Could you check a few things on this model? Use its own coordinates, in mm. A direction names the side the tool comes from. Give positions to 0.01 mm unless a question says otherwise; leave off trailing zeros. Order: outer loops, then holes, each group sorted by start corner. A loop starts at its lowest first (then second) coordinate and runs counter-clockwise, first axis right, second up. Notation, with made-up numbers: M -17.75,48.25 L 35.25,48.25 A13 cw 35.25,63.25 Z; hole C 54.5,48.25 d2. An arc over 180 degrees is marked long. Use a Markdown table: item, result. Add a question column.
```python
from build123d import *

# Parameters (mm, degrees)
SKETCH1_W           = 37
SKETCH1_H           = 37
BOSS_EXTRUDE1_DEPTH = 1220
SKETCH2_W           = 20
SKETCH2_H           = 20
SKETCH2_W_2         = 5
CUT_EXTRUDE1_DEPTH  = 50
CUT_EXTRUDE2_DEPTH  = 10
CUT_EXTRUDE3_DEPTH  = 10
SKETCH5_R           = 3
CUT_EXTRUDE4_DEPTH  = 1222.310771262


with BuildPart() as part:
    # Sketch1 → Boss-Extrude1 (new body)
    with BuildSketch(Plane(origin=(0, 0, 0), x_dir=(1, 0, 0), z_dir=(0, 1, 0))):
        with BuildLine():
            Line((0.5, 0), (39.5, 0))
            ThreePointArc((39.5, 0), (39.853553391, 0.146446609), (40, 0.5))
            Line((40, 0.5), (40, 39.5))
            ThreePointArc((40, 39.5), (39.853553391, 39.853553391), (39.5, 40))
            Line((39.5, 40), (0.5, 40))
            ThreePointArc((0.5, 40), (0.146446609, 39.853553391), (0, 39.5))
            Line((0, 39.5), (0, 0.5))
            ThreePointArc((0, 0.5), (0.146446609, 0.146446609), (0.5, 0))
        make_face()
        with Locations((20, 20)):
            Rectangle(SKETCH1_W, SKETCH1_H, mode=Mode.SUBTRACT)
    extrude(amount=BOSS_EXTRUDE1_DEPTH)

    # Sketch2 → Cut-Extrude1 (cut)
    with BuildSketch(Plane.XY):
        with Locations((10, 1210)):
            Rectangle(SKETCH2_W, SKETCH2_H)
        with Locations((37.5, 1210)):
            Rectangle(SKETCH2_W_2, SKETCH2_H)
        with Locations((10, 10)):
            Rectangle(SKETCH2_W, SKETCH2_H)
        with Locations((37.5, 10)):
            Rectangle(SKETCH2_W_2, SKETCH2_H)
    extrude(amount=-CUT_EXTRUDE1_DEPTH, mode=Mode.SUBTRACT)

    # Sketch3 → Cut-Extrude2 (cut)
    with BuildSketch(Plane.XY.offset(-40)):
        Polygon((30, 893.6), (20, 893.6), (20, 853.6), (30, 853.6), (30, 855.6), (22, 855.6), (22, 891.6), (30, 891.6), align=None)
        Polygon((20, 326.4), (20, 366.4), (30, 366.4), (30, 364.4), (22, 364.4), (22, 328.4), (30, 328.4), (30, 326.4), align=None)
    extrude(amount=CUT_EXTRUDE2_DEPTH, mode=Mode.SUBTRACT)

    # Sketch4 → Cut-Extrude3 (cut)
    with BuildSketch(Plane(origin=(0, 0, -40), x_dir=(-1, 0, 0), z_dir=(0, 0, -1))):
        Polygon((-30, 703.06), (-20, 703.06), (-20, 663.06), (-30, 663.06), (-30, 665.06), (-22, 665.06), (-22, 701.06), (-30, 701.06), align=None)
        Polygon((-30, 518.94), (-30, 516.94), (-20, 516.94), (-20, 556.94), (-30, 556.94), (-30, 554.94), (-22, 554.94), (-22, 518.94), align=None)
    extrude(amount=-CUT_EXTRUDE3_DEPTH, mode=Mode.SUBTRACT)

    # Sketch5 → Cut-Extrude4 (cut, through all)
    with BuildSketch(Plane(origin=(0, 0, -40), x_dir=(-1, 0, 0), z_dir=(0, 0, -1))):
        with Locations((-23, 1115.75)):
            Circle(SKETCH5_R)
        with Locations((-23, 945.75)):
            Circle(SKETCH5_R)
        with Locations((-23, 641)):
            Circle(SKETCH5_R)
        with Locations((-23, 579)):
            Circle(SKETCH5_R)
        with Locations((-23, 274.25)):
            Circle(SKETCH5_R)
        with Locations((-23, 104.25)):
            Circle(SKETCH5_R)
    extrude(amount=-CUT_EXTRUDE4_DEPTH, mode=Mode.SUBTRACT)


solid = part.part
```
1) We'd pull the mould along Z, two halves only. Please class faces 1 (the face through (20, 601, -40)), 2 (the face through (38.5, 602, -20)), 3 (the face through (40, 602, -20)): pulls with the +Z half, pulls with the -Z half, needs draft (parallel to the pull), parting line crosses it, or undercut.
2) For pin 1 (9.5 mm diameter, centred on x = 23, y = 641, fed in from -Z); pin 2 (5.5 mm diameter, centred on x = 23, y = 104.25, fed in from +Z); pin 3 (1.6 mm diameter, centred on y = 12, z = -0.5, fed in from -X); pin 4 (1.2 mm diameter, centred on y = 13, z = -39.5, fed in from +X), each with a flat end and sliding along its axis, tell me the tip position at first contact or that it passes through.
3) For faces 4 (the face through (0, 602, -20)), 5 (the face through (20, 601, -1.5)), 6 (the face through (1, 1200, -20)), 7 (the face through (1, 20, -20)), which set-ups out of +Z, -Z, +X, -X, +Y, -Y let a thin tool reach every point of the face, with its end or its side?
4) Suppose I cut it at B-B on y = 459. Please give me the cut outline in (x, z), and give its area (3 significant figures).
5) Suppose I cut it at A-A on x = 9.5. Please give me the cut outline in (y, z).
6) Suppose I cut it at C-C on z = -23. Please give me the cut outline in (x, y).
7) Please list where these lines run through material, in increasing order: line 1 (X direction, y = 686, z = -18); line 2 (Z direction, x = 26, y = 328.5). Write a range as from..to.
Values found:
| question | item | result |
|---|---|---|
| 1 | face 1 | pulls with the -Z half |
| 1 | face 2 | undercut |
| 1 | face 3 | needs draft |
| 2 | pin 1 | stops at z = -40 |
| 2 | pin 2 | passes through |
| 2 | pin 3 | stops at x = 20 |
| 2 | pin 4 | stops at x = 35 |
| 3 | face 4 | +Z, -Z, -X, +Y, -Y |
| 3 | face 5 | +Y, -Y |
| 3 | face 6 | +Z, -Z, -X, +Y |
| 3 | face 7 | +Z, -Z, -X, -Y |
| 4 | outline | M 0,-39.5 A0.5 ccw 0.5,-40 L 39.5,-40 A0.5 ccw 40,-39.5 L 40,-0.5 A0.5 ccw 39.5,0 L 0.5,0 A0.5 ccw 0,-0.5 Z; hole M 1.5,-38.5 L 38.5,-38.5 L 38.5,-1.5 L 1.5,-1.5 Z |
| 4 | area | 231 mm^2 |
| 5 | outline | M 20,-40 L 1200,-40 L 1200,-38.5 L 20,-38.5 Z; M 20,-1.5 L 1200,-1.5 L 1200,0 L 20,0 Z |
| 6 | outline | M 0,20 L 1.5,20 L 1.5,1200 L 0,1200 Z; M 38.5,20 L 40,20 L 40,1200 L 38.5,1200 Z |
| 7 | line 1 | x = 0..1.5, 38.5..40 |
| 7 | line 2 | z = -40..-38.5, -1.5..0 |
